Read the model definition and answer for the solid it produces. Units are mm, in the model's axes. Face numbers are marked on the shaded views. A direction names the side the tool comes from. Give positions to 0.01 mm unless a question says otherwise; leave off trailing zeros. Loops run counter-clockwise (first coordinate to the right, second up) from the corner with the lowest first, then second, coordinate; pieces in that order, holes last. Notation, with made-up numbers: (71.5, 62.25) - (102.5, 62.25) arc R26 cw to (102.5, 85.25) - close; hole circle Ø8 at (21.5, 2.5). An arc over 180 degrees is marked (long way). Use a Markdown table: item, result. Add a question column.
Item 1: A cutting plane is placed at C-C (x = -2). Determine the outline of the cut face in (y, z), plus the area to 3 significant figures.
Item 2: Consider probe 1 along Z at (x, y) = (-1.65, -6.5); probe 2 along Z at (x, y) = (-1.3, -6.5); probe 3 along Y at (x, z) = (-1.2, -10). Determine where each line is inside the solid, lowest interval first. Write a range as [from, to].
Item 3: Which of the six approach directions +Z, -Z, +X, -X, +Y, -Y give full straight-line access (tool end or side, diameter ignored) to the marked faces 1, 2 and 3?
Item 4: A cutting plane is placed at B-B (y = -6.5). Determine the outline of the cut face in (x, z), plus the area to 3 significant figures.
Item 5: A cutting plane is placed at A-A (z = -10). Determine the outline of the cut face in (x, y).
Item 6: Each of these flat-tipped pins is pushed along its axis until it touches: P1, Ø4.5, axis at x = -5.5, y = -9.5, coming from the +Z side; P2, Ø6.5, axis at y = -9.5, z = -10.5, coming from the -X side; P3, Ø1.2, axis at y = -4, z = -22.5, coming from the +X side; P4, Ø3, axis at y = -6.5, z = -10, coming from the +X side. Where does it stop, or does it pass through?
Item 7: A cutting plane is placed at D-D (y = -0.75). Determine the outline of the cut face in (x, z), plus the area to 3 significant figures.
Item 8: For a pull along Z with two mould halves and no side action, classify the marked faces 4, 5, 6 and 7 as +Z half, -Z half, draft (parallel to the pull), parting line (faces both ways), or undercut.
Autodesk Inventor part; units mm, degrees
ref_plane "YZ Plane" through (0, 0, 0) normal (1, 0, 0) x (0, 1, 0)
ref_plane "XZ Plane" through (0, 0, 0) normal (0, 1, 0) x (-1, 0, 0)
ref_plane "XY Plane" through (0, 0, 0) normal (0, 0, 1) x (1, 0, 0)
sketch "Sketch1" plane through (0, 0, 0) normal (0, 1, 0) x (-1, 0, 0)
  line L0 (0, 0) -> (3, 0)
  line L1 (3, 0) -> (3, -20)
  line L2 (3, -20) -> (0, -20)
  line L3 (0, -20) -> (0, 0)
  line L4 (3, -20) -> (16, -20)
  line L5 (16, -20) -> (16, -17)
  line L6 (16, -17) -> (3, -17)
  line L7 (3, -17) -> (3, -20)
  dimension "d0" = 3
  dimension "d1" = 20
  dimension "d2" = 13
  dimension "d3" = 3
extrude "Extrusion1" add sketch "Sketch1" against normal blind 13
sketch "Sketch2" plane through (0, 0, 0) normal (0, 1, 0) x (1, 0, 0)
  line L0 (-16, 20) -> (0, 20)
  line L1 (0, 0) -> (0, 20)
  line L2 (-6.3982, 20) -> (-3.3982, 20)
  line L3 (-3.3982, 20) -> (-3.3982, 22)
  line L4 (-3.3982, 22) -> (-6.3982, 22)
  line L5 (-6.3982, 22) -> (-6.3982, 20)
  line L6 (-6.3982, 20) -> (-3.3982, 22) construction
  line L7 (-6.3982, 22) -> (-3.3982, 20) construction
  line L8 (0, 20) -> (-16, 20)
  line L9 (-1.4593, 20) -> (-8.4593, 20)
  line L10 (-8.4593, 20) -> (-8.4593, 24)
  line L11 (-8.4593, 24) -> (-1.4593, 24)
  line L12 (-1.4593, 24) -> (-1.4593, 20)
  line L13 (-8.4593, 22) -> (-1.4593, 22)
  point P0 (-4.8982, 20)
  point P1 (-4.8982, 21)
  dimension "d6" = 4.8982
  dimension "d7" = 3
  dimension "d8" = 2
  dimension "d9" = 7
  dimension "d10" = 4
extrude "Extrusion2" add sketch "Sketch2" against normal up to surface (13 mm away) contours L5 L4 L3 L0
extrude "Extrusion3" add sketch "Sketch2" against normal blind 2
extrude "Extrusion4" add sketch "Sketch2" against normal up to surface (13 mm away) contours L10 L11 L12 L13 L4
fillet "Fillet1" radius 1.5 2 edges at (-6.3982, -13, -21) (-3.3982, -13, -21)
sketch "Sketch3" plane through (0, 0, 0) normal (0, 1, 0) x (1, 0, 0)
  line L0 (-16, 17) -> (-3, 17)
  line L1 (-8.4593, 20) -> (-16, 20)
  line L2 (-16, 17) -> (-8.4593, 17)
  line L3 (-8.4593, 17) -> (-8.4593, 20)
  line L4 (-8.4593, 20) -> (-16, 20)
  line L5 (-16, 20) -> (-16, 17)
  point P0 (0, 0)
extrude "Extrusion5" cut sketch "Sketch3" against normal up to next
sketch "Sketch7" plane through (-3, 0, -17) normal (-1, 0, 0) x (0, 0, 1)
  line L0 (0, 0) -> (17, 0)
  line L1 (17, 0) -> (17, -13)
  point P0 (7, -6.5)
  dimension "d41" = 6.5
  dimension "d42" = 10
hole "Hole2" at (-3, -6.5, -10) direction (1, 0, 0) diameter 4 end through all
properties part number "bloceur_alim"
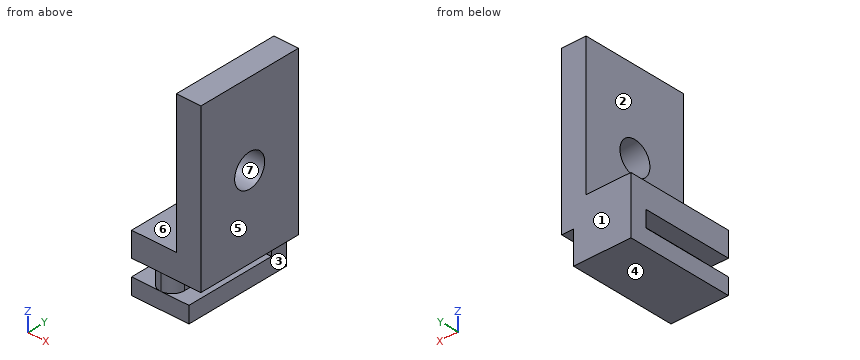
Geometry says:
| question | item | result |
|---|---|---|
| 1 | outline | (-13, -24) - (0, -24) - (0, 0) - (-13, 0) - (-13, -20) - (-2, -20) - (-2, -22) - (-13, -22) - close; hole circle Ø4 at (-6.5, -10) |
| 1 | area | 277 mm² |
| 2 | probe 1 | [-24, -22], [-20, -12], [-8, 0] |
| 2 | probe 2 | [-20, -12], [-8, 0] |
| 2 | probe 3 | [-13, -8.5], [-4.5, 0] |
| 3 | face 1 | +Z, -Z, +X, -X, +Y |
| 3 | face 2 | +Z, -X, +Y, -Y |
| 3 | face 3 | -Z, +X, +Y, -Y |
| 4 | outline | (-8.46, -24) - (-1.46, -24) - (-1.46, -22) - (-3.4, -22) - (-3.4, -20) - (0, -20) - (0, -12) - (-3, -12) - (-3, -17) - (-8.46, -17) - (-8.46, -20) - (-6.4, -20) - (-6.4, -22) - (-8.46, -22) - close; (-3, -8) - (0, -8) - (0, 0) - (-3, 0) - close |
| 4 | area | 84.4 mm² |
| 5 | outline | (-3, -13) - (0, -13) - (0, -8.5) - (-3, -8.5) - close; (-3, -4.5) - (0, -4.5) - (0, 0) - (-3, 0) - close |
| 6 | P1 | z = -17 |
| 6 | P2 | x = -3 |
| 6 | P3 | x = -1.46 |
| 6 | P4 | through |
| 7 | outline | (-8.46, -24) - (-1.46, -24) - (-1.46, -20) - (0, -20) - (0, 0) - (-3, 0) - (-3, -17) - (-8.46, -17) - close |
| 7 | area | 104 mm² |
| 8 | face 4 | -Z half |
| 8 | face 5 | draft |
| 8 | face 6 | +Z half |
| 8 | face 7 | undercut |
